Source: CAD feature listing. Evaluate the final solid. Frame: model axes, mm. A direction names the side the tool comes from. Round coordinates to 2 decimals unless told otherwise and drop trailing zeros. Write each loop counter-clockwise with the first axis right and the second up, starting at its lowest first coordinate (ties: lowest second). Pieces come first, ordered by that corner, then holes. Notation, with made-up numbers: (44, 15.25) - (62, 15.25) arc R33 cw to (62, 43.25) - close; hole circle Ø3 at (80, 88.25). An arc over 180 degrees is marked (long way). Write item = value, one per line. Start each with the question number.
```python
from build123d import *

# Parameters (mm, degrees)
ESQUISSE1_W        = 71
ESQUISSE1_H        = 28
BOSS_EXTRU_1_DEPTH = 168
BOSS_EXTRU_2_DEPTH = 2
ESQUISSE3_R        = 3
BOSS_EXTRU_3_DEPTH = 8


with BuildPart() as part:
    # Esquisse1 → Boss.-Extru.1 (new body)
    with BuildSketch(Plane(origin=(0, 0, 0), x_dir=(1, 0, 0), z_dir=(0, 1, 0))):
        Rectangle(ESQUISSE1_W, ESQUISSE1_H)
    extrude(amount=BOSS_EXTRU_1_DEPTH)

    # Esquisse2 → Boss.-Extru.2 (add)
    with BuildSketch(Plane(origin=(0, 168, 0), x_dir=(1, 0, 0), z_dir=(0, 1, 0))):
        with BuildLine():
            Line((-24.5, 4.5), (-14.5, 4.5))
            ThreePointArc((-14.5, 4.5), (-10, 0), (-14.5, -4.5))
            Line((-14.5, -4.5), (-24.5, -4.5))
            ThreePointArc((-24.5, -4.5), (-29, 0), (-24.5, 4.5))
        make_face()
        with BuildLine():
            Line((24.5, 4.5), (14.5, 4.5))
            ThreePointArc((14.5, 4.5), (10, 0), (14.5, -4.5))
            Line((14.5, -4.5), (24.5, -4.5))
            ThreePointArc((24.5, -4.5), (29, 0), (24.5, 4.5))
        make_face()
    extrude(amount=BOSS_EXTRU_2_DEPTH)

    # Esquisse3 → Boss.-Extru.3 (add)
    with BuildSketch(Plane(origin=(0, 170, 0), x_dir=(1, 0, 0), z_dir=(0, 1, 0))):
        with Locations((-19.5, 0)):
            Circle(ESQUISSE3_R)
        with Locations((19.5, 0)):
            Circle(ESQUISSE3_R)
    extrude(amount=BOSS_EXTRU_3_DEPTH)


solid = part.part
```
(1) Section D-D (x = 6). Return the cut outline in (y, z).
(2) Section B-B (x = -19.5). Return the cut outline in (y, z).
(3) Section C-C (z = 11.5). Return the cut outline in (x, y), plus the area to 3 significant figures.
(4) Ray query, L1, parallel to Y at x = -30, z = 6.5; L2, parallel to Y at x = 13.5, z = 1.25. Return the intervals inside material, ascending. Write a range as from..to.
(5) Contact query for flat-ended pins moving along their axis: P1, Ø0.6, axis at x = 20.5, y = 169, coming from the -Z side; P2, Ø2, axis at x = 17, y = 169.5, coming from the +Z side; P3, Ø14, axis at x = -9.5, z = 4.5, coming from the +Y side. Output: stop coordinate, or through.
(6) Reachability of faces 4 (the flat face through (0, 83, 14)), 5 (the cylindrical face through (-29, 169, 0)), 6 (the cylindrical face through (-10, 169, 0)) from +Z, -Z, +X, -X, +Y, -Y: full face, straight path, thin tool, end or side. Return the list, or none.
(7) Pull-direction query (X, two-part tool) for faces 1 (the cylindrical face through (29, 169, 0)), 2 (the flat face through (-35.5, 83, 0)), 3 (the flat face through (17, 170, -2)); classes: +X half, -X half, draft (parallel to the pull), parting line (faces both ways), or undercut.
(8) Section A-A (z = 0). Return the cut outline in (x, y), plus the area to 3 significant figures.
Solution:
q1.outline = (0, -14) - (168, -14) - (168, 14) - (0, 14) - close
q2.outline = (0, -14) - (168, -14) - (168, -4.5) - (170, -4.5) - (170, -3) - (178, -3) - (178, 3) - (170, 3) - (170, 4.5) - (168, 4.5) - (168, 14) - (0, 14) - close
q3.outline = (-35.5, 0) - (35.5, 0) - (35.5, 168) - (-35.5, 168) - close
q3.area = 11,900 mm^2
q4.L1 = 0..168
q4.L2 = 0..170
q5.P1 = -4.5
q5.P2 = 4.5
q5.P3 = 170
q6.face_4 = +Z, +X, -X, +Y, -Y
q6.face_5 = -X, +Y
q6.face_6 = +Y
q7.face_1 = +X half
q7.face_2 = -X half
q7.face_3 = undercut
q8.outline = (-35.5, 0) - (35.5, 0) - (35.5, 168) - (29, 168) - (29, 170) - (22.5, 170) - (22.5, 178) - (16.5, 178) - (16.5, 170) - (10, 170) - (10, 168) - (-10, 168) - (-10, 170) - (-16.5, 170) - (-16.5, 178) - (-22.5, 178) - (-22.5, 170) - (-29, 170) - (-29, 168) - (-35.5, 168) - close
q8.area = 12,100 mm^2
